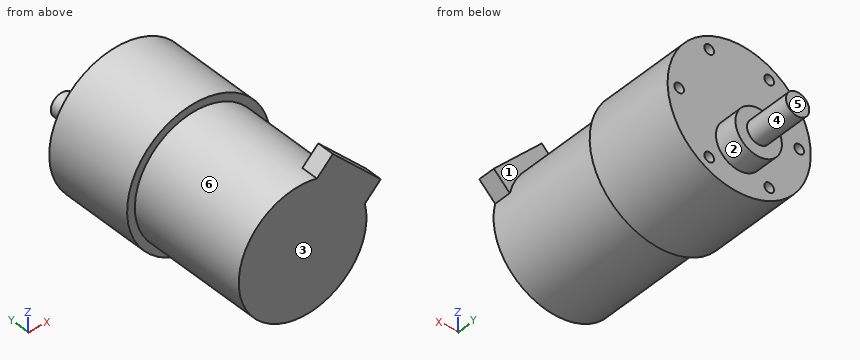
from build123d import *

# Parameters (mm, degrees)
SKETCH_1_R             = 16.5
EXTRUDE_1_DEPTH        = 32
SKETCH_2_R             = 18.5
EXTRUDE_2_DEPTH        = 24
SKETCH_3_R             = 6
EXTRUDE_3_DEPTH        = 6
SKETCH_4_R             = 3
EXTRUDE_4_DEPTH        = 12
HOLE_WIZARD_M3_1_D     = 2.5
HOLE_WIZARD_M3_1_DEPTH = 3.3
HOLE_WIZARD_M3_1_TIP   = 0.751075774
EXTRUDE_5_DEPTH        = 4.5


with BuildPart() as part:
    # 草图1 → 凸台-拉伸1 (new body)
    with BuildSketch(Plane(origin=(0, 0, 0), x_dir=(1, 0, 0), z_dir=(0, 1, 0))):
        with Locations(Location((0, 0, 0), (0, 0, 270))):
            Circle(SKETCH_1_R)
    extrude(amount=EXTRUDE_1_DEPTH)

    # 草图2 → 凸台-拉伸2 (add)
    with BuildSketch(Plane(origin=(0, 32, 0), x_dir=(1, 0, 0), z_dir=(0, 1, 0))):
        with Locations(Location((0, 0, 0), (0, 0, 270))):
            Circle(SKETCH_2_R)
    extrude(amount=EXTRUDE_2_DEPTH)

    # 草图3 → 凸台-拉伸3 (add)
    with BuildSketch(Plane(origin=(0, 56, 0), x_dir=(1, 0, 0), z_dir=(0, 1, 0))):
        with Locations(Location((0, 7, 0), (0, 0, 270))):
            Circle(SKETCH_3_R)
    extrude(amount=EXTRUDE_3_DEPTH)

    # 草图4 → 凸台-拉伸4 (add)
    with BuildSketch(Plane(origin=(0, 62, 0), x_dir=(1, 0, 0), z_dir=(0, 1, 0))):
        with Locations(Location((0, 7, 0), (0, 0, 270))):
            Circle(SKETCH_4_R)
    extrude(amount=EXTRUDE_4_DEPTH)

    # M3 螺纹孔的螺纹孔钻头1
    with Locations(Plane(origin=(0, 56, 0), x_dir=(1, 0, 0), z_dir=(0, 1, 0))):
        with Locations((-7.75, 13.423393759), (7.75, 13.423393759), (15.5, 0), (7.75, -13.423393759), (-7.75, -13.423393759), (-15.5, 0)):
            Hole(HOLE_WIZARD_M3_1_D / 2, depth=HOLE_WIZARD_M3_1_DEPTH)
            with Locations((0, 0, -(HOLE_WIZARD_M3_1_DEPTH + HOLE_WIZARD_M3_1_TIP / 2))):  # 118° drill point
                Cone(0, HOLE_WIZARD_M3_1_D / 2, HOLE_WIZARD_M3_1_TIP, mode=Mode.SUBTRACT)

    # 草图8 → 凸台-拉伸5 (add)
    with BuildSketch(Plane.XZ):
        Polygon((3.704415636, 16.078784307), (16.078784307, 3.704415636), (20.187898603, 7.813529932), (7.813529932, 20.187898603), align=None)
    extrude(amount=-EXTRUDE_5_DEPTH)


solid = part.part
Can you work these out from the model? Positions are in its coordinate system, mm. Face numbers are marked on the shaded views. A direction names the side the tool comes from. Coordinates: 2 decimals unless noted, no trailing zeros. Write each loop counter-clockwise with the first axis right and the second up, starting at its lowest first coordinate (ties: lowest second). Pieces come first, ordered by that corner, then holes. Notation, with made-up numbers: (-28, -18) -> (-2, -18) arc R24 ccw to (-2, 14) -> close; hole circle Ø6 at (-37, 13.5). An arc over 180 degrees is marked (long way). Write each question's results on one line, items separated by ' | '. Start each with the question number.
Q1. Imagine slicing it at D-D (x = 10.5). Write out the boundary of the cut face in (y, z).
Q2. Imagine slicing it at B-B (z = 9.5). Write out the boundary of the cut face in (x, y).
Q3. Imagine slicing it at A-A (x = 0). Write out the boundary of the cut face in (y, z), then the cut area to 3 significant figures.
Q4. On a 3-axis mill with a long thin cutter (end or side, diameter ignored), from which of +Z, -Z, +X, -X, +Y, -Y can I reach the whole of each face in a straight line? I mean the marked faces 1, 2 and 3. Say none if no direction works.
Q5. If I drill on probe 1 along Y at (x, z) = (16, 4.5); probe 2 along Z at (x, y) = (7, 54); probe 3 along Z at (x, y) = (7.75, 53.7), over which ranges is the centre line in solid material (lowest first)?
Q6. Imagine slicing it at C-C (y = 29.5). Write out the boundary of the cut face in (x, z).
Q7. We'd pull the mould along Y, two halves only. Please class the marked faces 4, 5 and 6: +Y half, -Y half, draft (parallel to the pull), parting line (faces both ways), or undercut.
Q8. I'm going to push flat-ended pins straight in: pin 1 (4 mm diameter, centred on x = 7.75, z = -13.42, fed in from +Y); pin 2 (1 mm diameter, centred on x = -4, z = -2.5, fed in from +Y); pin 3 (10 mm diameter, centred on x = 15.5, y = 52.5, fed in from +Z). Where does each tip first touch, or does it pass through?
Taken from the geometry:
1) outline: (0, -12.73) -> (32, -12.73) -> (32, -15.23) -> (56, -15.23) -> (56, 15.23) -> (32, 15.23) -> (32, 12.73) -> (4.5, 12.73) -> (4.5, 17.5) -> (0, 17.5) -> close
2) outline: (-15.87, 32) -> (-13.49, 32) -> (-13.49, 0) -> (18.5, 0) -> (18.5, 4.5) -> (13.49, 4.5) -> (13.49, 32) -> (15.87, 32) -> (15.87, 56) -> (-15.87, 56) -> close
3) outline: (0, -16.5) -> (32, -16.5) -> (32, -18.5) -> (56, -18.5) -> (56, -13) -> (62, -13) -> (62, -10) -> (74, -10) -> (74, -4) -> (62, -4) -> (62, -1) -> (56, -1) -> (56, 18.5) -> (32, 18.5) -> (32, 16.5) -> (0, 16.5) -> close | area: 2,090 mm^2
4) face 1: +Z, +X | face 2: +Y | face 3: +Z, -Z, +X, -X, -Y
5) probe 1: y = 0 to 4.5, 32 to 56 | probe 2: z = -17.12 to -14.42, -12.42 to 12.42, 14.42 to 17.12 | probe 3: z = -16.8 to -14.67, -12.17 to 12.17, 14.67 to 16.8
6) outline: circle Ø33 at (0, 0)
7) face 4: draft | face 5: +Y half | face 6: undercut
8) pin 1: stops at y = 56 | pin 2: stops at y = 62 | pin 3: stops at z = 15.23
